```python
from build123d import *

# Parameters (mm, degrees)
F0_W     = 80
F0_H     = 60
F1_DEPTH = 15
F3_DEPTH = 15


with BuildPart() as f1:
    # F0 (on Front) → F1 (new body)
    with BuildSketch(Plane.XZ):
        with Locations((40, 30)):
            Rectangle(F0_W, F0_H)
    extrude(amount=F1_DEPTH)

    # F2 (on Front) → F3 (join)
    with BuildSketch(Plane.XZ):
        Polygon((0, 30), (0, 0), (55, 0), (55, 60), (30, 60), (30, 30), align=None)
    extrude(amount=-F3_DEPTH)


solid = f1.part
```
Part model, mm, in its own coordinate system. A direction names the side the tool comes from. Give positions to 0.01 mm unless a question says otherwise; leave off trailing zeros. Order: outer loops, then holes, each group sorted by start corner. A loop starts at its lowest first (then second) coordinate and runs counter-clockwise, first axis right, second up. Notation, with made-up numbers: M 66,29 L 112,29 A21 cw 112,57 Z; hole C 73.25,5 d9. An arc over 180 degrees is marked long. Use a Markdown table: item, result. Add a question column.
(1) Drop flat-ended pins along their axis: P1, Ø12, axis at y = 7, z = 44.5, coming from the +X side; P2, Ø4.5, axis at x = 18, y = 7, coming from the +Z side; P3, Ø1.5, axis at y = 1.5, z = 32, coming from the -X side. Give the stop position or say it passes through.
(2) Saw through at A-A, the plane x = 23. Give the cut face in (y, z), and give its area (3 significant figures).
(3) Saw through at D-D, the plane x = 63. Give the cut face in (y, z).
(4) Saw through at B-B, the plane y = 3. Give the cut face in (x, z).
(5) Probe line 1 along X through (y, z) = (3.25, 44); line 2 along Y through (x, z) = (76.5, 3.5); line 3 along Z through (x, y) = (25, 8.25). List the from-to ranges inside material, lowest first. Write a range as [from, to].
(6) 3-axis set-ups, long thin cutter, end or side, ignore diameter. For faces 4 (the face through (33, 15, 24)), 5 (the face through (67, 0, 30)), 6 (the face through (15, 7, 30)): which of +Z, -Z, +X, -X, +Y, -Y reach the whole face in a straight line?
(7) Mould opens along X. For faces 1 (the face through (80, -7, 30)), 2 (the face through (31, 0, 0)), 3 (the face through (30, 7, 45)) say: +X half, -X half, draft (parallel to the pull), parting line (faces both ways), or undercut.
(8) Saw through at C-C, the plane z = 48.5. Give the cut face in (x, y), and give its area (4 significant figures).
Answer key:
| question | item | result |
|---|---|---|
| 1 | P1 | x = 55 |
| 1 | P2 | z = 30 |
| 1 | P3 | x = 30 |
| 2 | outline | M -15,0 L 15,0 L 15,30 L 0,30 L 0,60 L -15,60 Z |
| 2 | area | 1,350 mm^2 |
| 3 | outline | M -15,0 L 0,0 L 0,60 L -15,60 Z |
| 4 | outline | M 0,0 L 55,0 L 55,60 L 30,60 L 30,30 L 0,30 Z |
| 5 | line 1 | [30, 55] |
| 5 | line 2 | [-15, 0] |
| 5 | line 3 | [0, 30] |
| 6 | face 4 | +Z, -Z, +X, -X, +Y |
| 6 | face 5 | +Z, -Z, +X, +Y |
| 6 | face 6 | +Z, -X, +Y |
| 7 | face 1 | +X half |
| 7 | face 2 | draft |
| 7 | face 3 | -X half |
| 8 | outline | M 0,-15 L 80,-15 L 80,0 L 55,0 L 55,15 L 30,15 L 30,0 L 0,0 Z |
| 8 | area | 1,575 mm^2 |
